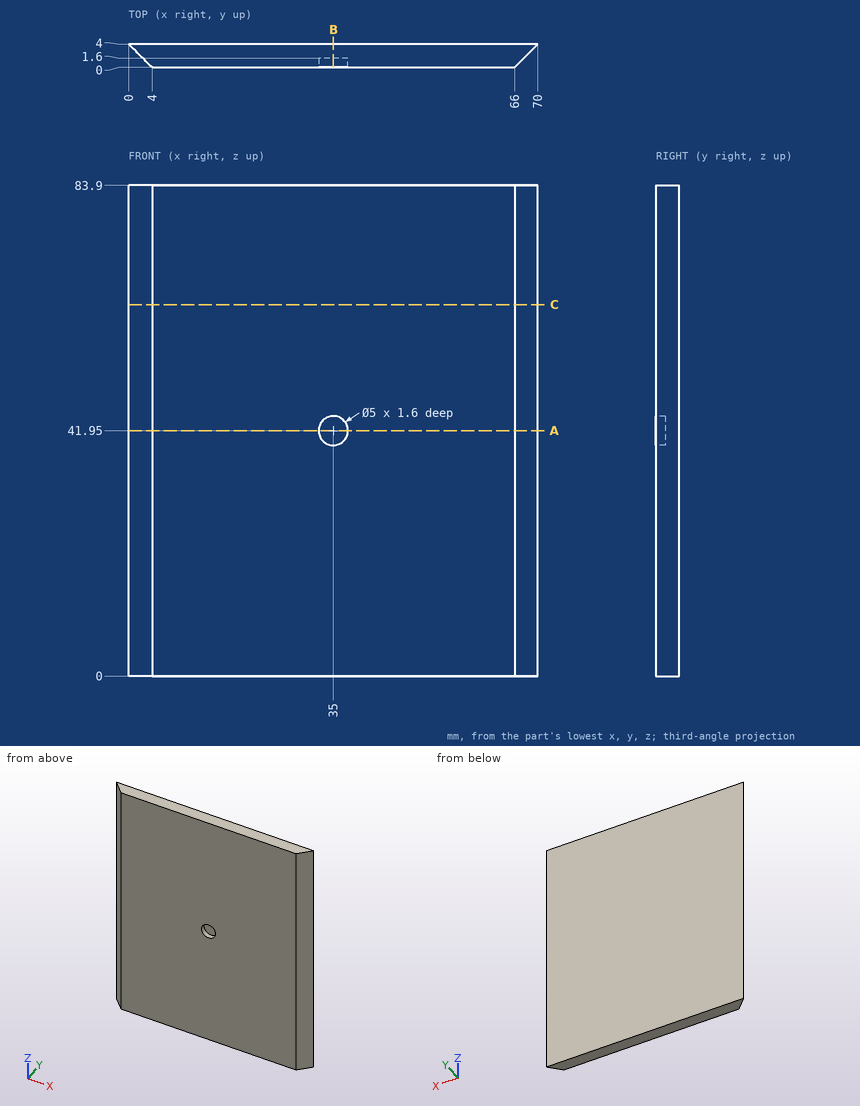
Geometry check sheet. Reference: drawing and pictorial views, mm from the part's lowest x, y, z. Give positions to 0.01 mm unless a question says otherwise; leave off trailing zeros. Order: outer loops, then holes, each group sorted by start corner. A loop starts at its lowest first (then second) coordinate and runs counter-clockwise, first axis right, second up. Notation, with made-up numbers: (77, 76.25) - (113, 76.25) arc R16 cw to (113, 82.25) - close; hole circle Ø10 at (45, 69.5). An arc over 180 degrees is marked (long way). Answer as CSV lines item,"result". Start each with the question number.
Item 1: Section check A-A, the plane z = 41.95. Record the boundary of the cut face in (x, y), plus the area to 3 significant figures.
Item 2: Section check B-B, the plane x = 35. Record the boundary of the cut face in (y, z), plus the area to 3 significant figures.
Item 3: Gauge pin test, flat end, axial feed: pin 1 (4 mm diameter, centred on x = 34, z = 43, fed in from -Y). Record the tip position at first contact, or that the pin passes through.
Item 4: Material ranges on L1, parallel to Z at x = 35, y = 0.6; L2, parallel to X at y = 1.45, z = 62; L3, parallel to X at y = 0.7, z = 52, recorded low to high.
Item 5: Section check C-C, the plane z = 63.5. Record the boundary of the cut face in (x, y).
Filled in:
1,outline,"(0, 4) - (4, 0) - (32.5, 0) - (32.5, 1.6) - (37.5, 1.6) - (37.5, 0) - (66, 0) - (70, 4) - close"
1,area,"256 mm^2"
2,outline,"(0, 0) - (4, 0) - (4, 83.9) - (0, 83.9) - (0, 44.45) - (1.6, 44.45) - (1.6, 39.45) - (0, 39.45) - close"
2,area,"328 mm^2"
3,pin 1,"y = 0"
4,L1,"0 to 39.45, 44.45 to 83.9"
4,L2,"2.55 to 67.45"
4,L3,"3.3 to 66.7"
5,outline,"(0, 4) - (4, 0) - (66, 0) - (70, 4) - close"
